Source: three-view drawing plus pictorial views. Frame: mm from the lowest corner of the part. A direction names the side the tool comes from. Give positions to 0.01 mm unless a question says otherwise; leave off trailing zeros. Loops run counter-clockwise (first coordinate to the right, second up) from the corner with the lowest first, then second, coordinate; pieces in that order, holes last. Notation, with made-up numbers: (39.25, -34) - (81.25, -34) arc R13 ccw to (81.25, -12) - close; hole circle Ø8 at (10, 41.25). An arc over 180 degrees is marked (long way). Answer in a Markdown table with one row per item.
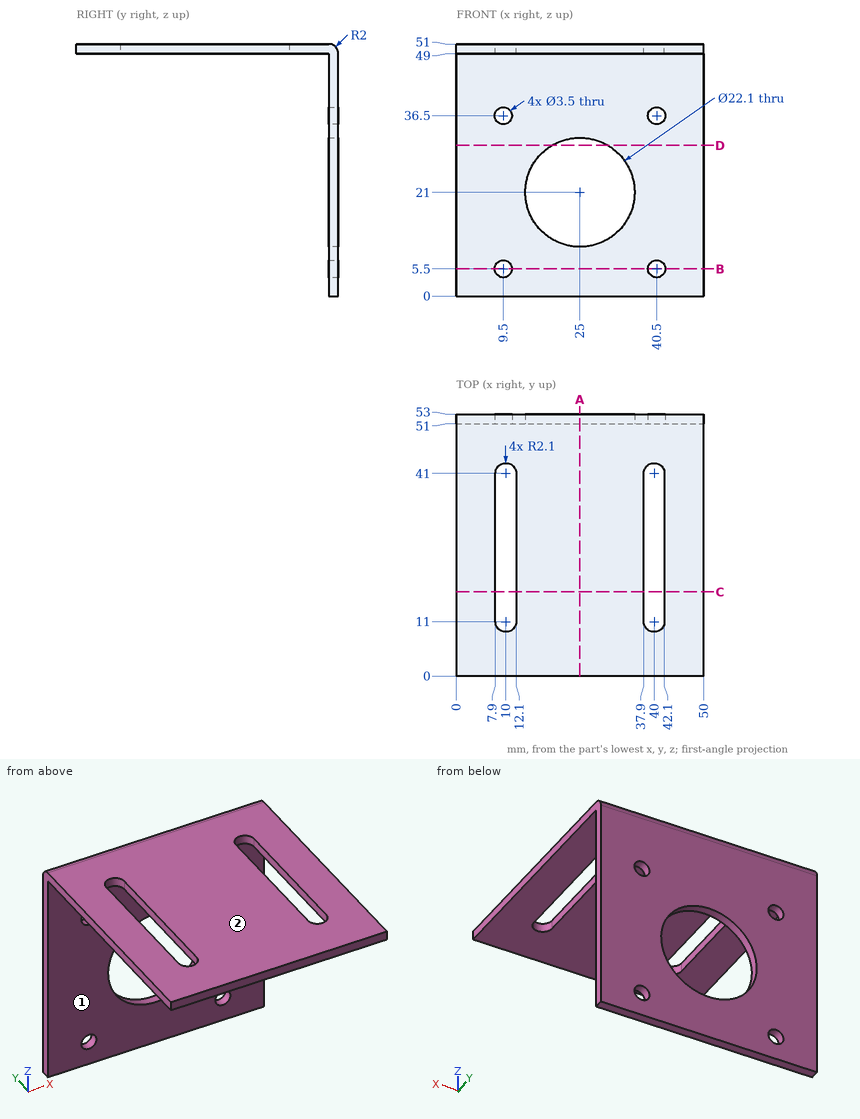
Q1. Cut plane B-B (z = 5.5). Output: boundary loops of the cut face in (x, y), and give its area (3 significant figures).
Check values:
| item | result |
|---|---|
| outline | (0, 51) - (7.75, 51) - (7.75, 53) - (0, 53) - close; (11.25, 51) - (38.75, 51) - (38.75, 53) - (11.25, 53) - close; (42.25, 51) - (50, 51) - (50, 53) - (42.25, 53) - close |
| area | 86.0 mm² |
Q2. Material intervals for line 1 along Z through (x, y) = (24.5, 3.5); line 2 along Z through (x, y) = (40, 52); line 3 along X through (y, z) = (52, 21), sorted ascending.
Check values:
| item | result |
|---|---|
| line 1 | 49 to 51 |
| line 2 | 0 to 3.82, 7.18 to 34.82, 38.18 to 50.73 |
| line 3 | 0 to 13.95, 36.05 to 50 |
Q3. Cut plane C-C (y = 17). Output: boundary loops of the cut face in (x, z).
Check values:
| item | result |
|---|---|
| outline | (0, 49) - (7.9, 49) - (7.9, 51) - (0, 51) - close; (12.1, 49) - (37.9, 49) - (37.9, 51) - (12.1, 51) - close; (42.1, 49) - (50, 49) - (50, 51) - (42.1, 51) - close |
Q4. Cut plane D-D (z = 30.5). Output: boundary loops of the cut face in (x, y).
Check values:
| item | result |
|---|---|
| outline | (0, 51) - (19.36, 51) - (19.36, 53) - (0, 53) - close; (30.64, 51) - (50, 51) - (50, 53) - (30.64, 53) - close |
Q5. First-contact query: pin 1 (1.6 mm diameter, centred on y = 24.5, z = 50, fed in from -X); pin 2 (4 mm diameter, centred on x = 40.5, z = 5.5, fed in from -Y); pin 3 (20 mm diameter, centred on x = 25, z = 21, fed in from -Y); pin 4 (3 mm diameter, centred on x = 45, y = 43, fed in from -Z). Flat tips, straight axial feed; report the tip coordinate or a pass-through.
Check values:
| item | result |
|---|---|
| pin 1 | x = 0 |
| pin 2 | y = 51 |
| pin 3 | through |
| pin 4 | z = 49 |
Q6. Reachability of the marked faces 1 and 2 from +Z, -Z, +X, -X, +Y, -Y: full face, straight path, thin tool, end or side. Return the list, or none.
Check values:
| item | result |
|---|---|
| face 1 | -Z, +X, -X, -Y |
| face 2 | +Z, +X, -X, +Y, -Y |
Q7. Cut plane A-A (x = 25). Output: boundary loops of the cut face in (y, z), and give its area (3 significant figures).
Check values:
| item | result |
|---|---|
| outline | (0, 49) - (51, 49) - (51, 32.05) - (53, 32.05) - (53, 49) arc R2 ccw to (51, 51) - (0, 51) - close; (51, 0) - (53, 0) - (53, 9.95) - (51, 9.95) - close |
| area | 159 mm² |
